```python
from build123d import *

# Parameters (mm, degrees)
SKETCH_1_W      = 21.5
SKETCH_1_H      = 20.2
EXTRUDE_1_DEPTH = 0.78
SKETCH_2_W      = 6.5
SKETCH_2_H      = 6.5
EXTRUDE_2_DEPTH = 1.5
SKETCH_3_W      = 8
SKETCH_3_H      = 8
EXTRUDE_3_DEPTH = 2.5
SKETCH_4_R      = 4
EXTRUDE_4_DEPTH = 2.8
SKETCH_5_W      = 15.5
SKETCH_5_H      = 11
EXTRUDE_5_DEPTH = 2.28


with BuildPart() as part:
    # Эскиз1 → Бобышка-Вытянуть1 (new body)
    with BuildSketch(Plane(origin=(0, 0, 0), x_dir=(1, 0, 0), z_dir=(0, 1, 0))):
        Rectangle(SKETCH_1_W, SKETCH_1_H)
    extrude(amount=EXTRUDE_1_DEPTH)

    # Эскиз2 → Бобышка-Вытянуть2 (add)
    with BuildSketch(Plane(origin=(0, 0.78, 0), x_dir=(1, 0, 0), z_dir=(0, 1, 0))):
        Rectangle(SKETCH_2_W, SKETCH_2_H)
    extrude(amount=EXTRUDE_2_DEPTH)

    # Эскиз3 → Бобышка-Вытянуть3 (add)
    with BuildSketch(Plane(origin=(0, 2.28, 0), x_dir=(1, 0, 0), z_dir=(0, 1, 0))):
        Rectangle(SKETCH_3_W, SKETCH_3_H)
    extrude(amount=EXTRUDE_3_DEPTH)

    # Эскиз4 → Бобышка-Вытянуть4 (add)
    with BuildSketch(Plane(origin=(0, 4.78, 0), x_dir=(1, 0, 0), z_dir=(0, 1, 0))):
        with Locations(Location((0, 0, 0), (0, 0, 270))):
            Circle(SKETCH_4_R)
    extrude(amount=EXTRUDE_4_DEPTH)

    # Эскиз5 → Бобышка-Вытянуть5 (add)
    with BuildSketch(Plane.XZ):
        with Locations((-4.5, -4.5)):
            Rectangle(SKETCH_5_W, SKETCH_5_H)
    extrude(amount=EXTRUDE_5_DEPTH)


solid = part.part
```
Could you check a few things on this model? Use its own coordinates, in mm. A direction names the side the tool comes from. Coordinates: 2 decimals unless noted, no trailing zeros. Order: outer loops, then holes, each group sorted by start corner. A loop starts at its lowest first (then second) coordinate and runs counter-clockwise, first axis right, second up. Notation, with made-up numbers: M 41.5,-32.75 L 69.5,-32.75 A30 cw 69.5,6.25 Z; hole C 42,17 d9. An arc over 180 degrees is marked long. Use one line per item in the form item = value. Start each with the question number.
1. Suppose I cut it at A-A on x = -8.75. Write out the boundary of the cut face in (y, z), then the cut area to 3 significant figures.
2. Suppose I cut it at D-D on z = -1.75. Write out the boundary of the cut face in (x, y).
3. Please list where these lines run through material, in increasing order: line 1 (Y direction, x = 3.5, z = 3.5); line 2 (X direction, y = 1.5, z = 1.5); line 3 (Y direction, x = -10, z = -4.5).
4. Suppose I cut it at C-C on y = 3.5. Write out the boundary of the cut face in (x, z).
5. Suppose I cut it at B-B on z = -5. Write out the boundary of the cut face in (x, y).
6. On a 3-axis mill with a long thin cutter (end or side, diameter ignored), from which of +Z, -Z, +X, -X, +Y, -Y can I reach the whole of each face in a straight line? I mean faces 4 (the cylindrical face through (-3.905, 6.16, -0.867)), 5 (the flat face through (0, 2, -3.25)), 6 (the flat face through (-4, 4, 0)), 7 (the flat face through (0, 2, 3.25)). Say none if no direction works.
7. For pin 1 (0.7 mm diameter, centred on x = -4.5, y = -1, fed in from -Z); pin 2 (0.8 mm diameter, centred on x = -11.5, z = -4.5, fed in from +Y); pin 3 (0.5 mm diameter, centred on x = 0.5, y = 1.5, fed in from -Z), each with a flat end and sliding along its axis, tell me the tip position at first contact or that it passes through.
8. We'd pull the mould along Y, two halves only. Please class faces 1 (the flat face through (-3, 4.78, -3)), 2 (the flat face through (-5, -1, 1)), 3 (the flat face through (3.25, 2, 0)): +Y half, -Y half, draft (parallel to the pull), parting line (faces both ways), or undercut.
Geometry says:
q1.outline = M -2.28,-10 L 0,-10 L 0,-10.1 L 0.78,-10.1 L 0.78,10.1 L 0,10.1 L 0,1 L -2.28,1 Z
q1.area = 40.8 mm^2
q2.outline = M -12.25,-2.28 L 3.25,-2.28 L 3.25,0 L 10.75,0 L 10.75,0.78 L 3.25,0.78 L 3.25,2.28 L 4,2.28 L 4,4.78 L 3.6,4.78 L 3.6,7.58 L -3.6,7.58 L -3.6,4.78 L -4,4.78 L -4,2.28 L -3.25,2.28 L -3.25,0.78 L -10.75,0.78 L -10.75,0 L -12.25,0 Z
q3.line_1 = 0 to 0.78, 2.28 to 4.78
q3.line_2 = -3.25 to 3.25
q3.line_3 = -2.28 to 0.78
q4.outline = M -4,-4 L 4,-4 L 4,4 L -4,4 Z
q5.outline = M -12.25,-2.28 L 3.25,-2.28 L 3.25,0 L 10.75,0 L 10.75,0.78 L -10.75,0.78 L -10.75,0 L -12.25,0 Z
q6.face_4 = +Y
q6.face_5 = -Z, +X, -X
q6.face_6 = +Z, -Z, -X, +Y
q6.face_7 = +Z, +X, -X
q7.pin_1 = -10
q7.pin_2 = 0
q7.pin_3 = -3.25
q8.face_1 = +Y half
q8.face_2 = draft
q8.face_3 = undercut
